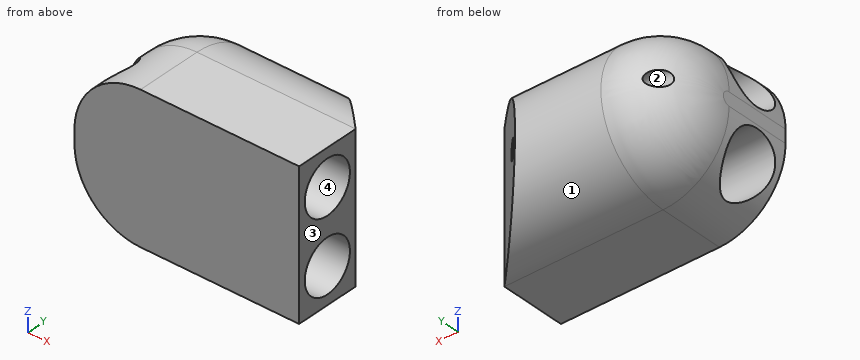
```python
from build123d import *

# Parameters (mm, degrees)
SKETCH1_W              = 21.59
SKETCH1_H              = 13.97
DEPTH_A_DEPTH          = 6.35
ROUND_EXTRUDE_DEPTH    = 21.59
ANGLE_CUT_DEPTH        = 29.967416609
STRING_HOLE_R          = 0.762
STRING_HOLE_CUT_DEPTH  = 29.967416609
ELASTIC_HOLES_R        = 2.54
ELASTIC_HOLE_CUT_DEPTH = 29.967416609
FILLET1_R              = 6.35


with BuildPart() as part:
    # Sketch1 → depth a (new body)
    with BuildSketch(Plane(origin=(0, 0, 0), x_dir=(1, 0, 0), z_dir=(0, 1, 0))):
        with Locations((-10.795, 6.985)):
            Rectangle(SKETCH1_W, SKETCH1_H)
    extrude(amount=DEPTH_A_DEPTH)

    # Sketch4 → round extrude (add)
    with BuildSketch(Plane(origin=(0, 0, 0), x_dir=(0, 0, -1), z_dir=(1, 0, 0))):
        with BuildLine():
            Line((0, 6.35), (13.97, 6.35))
            ThreePointArc((13.97, 6.35), (6.985, 13.335), (0, 6.35))
        make_face()
    extrude(amount=-ROUND_EXTRUDE_DEPTH)

    # Sketch5 → angle cut (cut, through all)
    with BuildSketch(Plane.XY):
        Polygon((0, 6.35), (0, 13.335), (-6.985, 13.335), align=None)
    extrude(amount=-ANGLE_CUT_DEPTH, mode=Mode.SUBTRACT)

    # string hole → string hole cut (cut, through all)
    with BuildSketch(Plane(origin=(0, 0, 0), x_dir=(0, 0, -1), z_dir=(1, 0, 0))):
        with Locations((6.985, 11.684)):
            Circle(STRING_HOLE_R)
    extrude(amount=-STRING_HOLE_CUT_DEPTH, mode=Mode.SUBTRACT)

    # elastic holes → elastic hole cut (cut, through all)
    with BuildSketch(Plane(origin=(0, 0, 0), x_dir=(0, 0, -1), z_dir=(1, 0, 0))):
        with Locations((3.4925, 3.175)):
            Circle(ELASTIC_HOLES_R)
        with Locations(Location((10.4775, 3.175, 0), (0, 0, 180))):
            Circle(ELASTIC_HOLES_R)
    extrude(amount=-ELASTIC_HOLE_CUT_DEPTH, mode=Mode.SUBTRACT)

    # Fillet1
    # the kernel refuses this fillet: 6.35 mm, written as the material it takes off along each edge
    with BuildSketch(Plane(origin=(-21.59, 6.35, -6.985), x_dir=(0, 0, -1), z_dir=(0, -1, 0))) as fillet1_piece_1:
        with BuildLine():
            CenterArc((6.985 - FILLET1_R, FILLET1_R), FILLET1_R, 270, 90)
            Line((6.985, FILLET1_R), (6.985, 0))
            Line((6.985, 0), (6.985 - FILLET1_R, 0))
        make_face()
    revolve(axis=Axis((-21.59, 6.35, -6.985), (1, 0, 0)), revolution_arc=180, mode=Mode.SUBTRACT)
    with BuildSketch(Plane(origin=(-21.59, -15.875, 0), x_dir=(1, 0, 0), z_dir=(0, 1, 0)), Plane(origin=(-21.59, -15.875, -13.97), x_dir=(0, 0, 1), z_dir=(0, 1, 0))) as fillet1_piece_2:
        with BuildLine():
            CenterArc((FILLET1_R, FILLET1_R), FILLET1_R, 180, 90)
            Line((0, FILLET1_R), (0, 0))
            Line((0, 0), (FILLET1_R, 0))
        make_face()
    extrude(amount=22.225, mode=Mode.SUBTRACT)


solid = part.part
```
Could you check a few things on this model? Use its own coordinates, in mm. Face numbers are marked on the shaded views. Round coordinates to 2 decimals unless told otherwise and drop trailing zeros. Write each loop counter-clockwise with the first axis right and the second up, starting at its lowest first coordinate (ties: lowest second). Pieces come first, ordered by that corner, then holes. Notation, with made-up numbers: M 78,-6.75 L 116,-6.75 A19 cw 116,28.25 Z; hole C 83.5,0 d6. An arc over 180 degrees is marked long. Answer in a Markdown table with one row per item. Add a question column.
Q1. Imagine slicing it at B-B (x = -13.75). Give the number of separate pieces and of enclosed holes in the cut face, then the cut area to 3 significant figures.
Q2. Imagine slicing it at A-A (y = 4.75). Please give me the cut outline in (x, z).
Q3. Will these pins go through, and if not, where does the flat tip stop? pin 1 Ø5 at (y, z) = (10.5, -2.5) entering from -X; pin 2 Ø1.5 at (x, y) = (-9.5, 10.5) entering from +Z; pin 3 Ø3 at (x, z) = (-19, -8.5) entering from +Y.
Q4. If I drill on line 1 (Z direction, x = -15.5, y = 2); line 2 (Z direction, x = -8.5, y = 1); line 3 (Y direction, x = -8.75, z = -3.75), over which ranges is the centre line in solid material (lowest first)? Write a range as from..to.
Q5. If we mould it in two halves opening along Y, with no side actions, what happens to the marked faces 1, 2, 3 and 4? For each: +Y half, -Y half, draft (parallel to the pull), parting line (faces both ways), or undercut.
Values:
| question | item | result |
|---|---|---|
| 1 | separate pieces | 1 |
| 1 | enclosed holes | 3 |
| 1 | area | 123 mm^2 |
| 2 | outline | M -21.59,-7.62 A6.35 ccw -21.53,-8.48 L 0,-8.48 L 0,-5.49 L -21.53,-5.49 A6.35 ccw -21.59,-6.35 Z; M -19.34,-12.47 A6.35 ccw -15.24,-13.97 L 0,-13.97 L 0,-12.47 Z; M -19.34,-1.5 L 0,-1.5 L 0,0 L -15.24,0 A6.35 ccw Z |
| 3 | pin 1 | x = -20.85 |
| 3 | pin 2 | z = -0.88 |
| 3 | pin 3 | y = 12.81 |
| 4 | line 1 | -13.96..-12.73, -8.23..-5.74, -1.24..-0.01 |
| 4 | line 2 | -13.97..-11.79, -9.17..-4.8, -2.18..0 |
| 4 | line 3 | 0..0.65, 5.7..12.54 |
| 5 | face 1 | +Y half |
| 5 | face 2 | undercut |
| 5 | face 3 | draft |
| 5 | face 4 | undercut |
